Source: CAD feature listing. Evaluate the final solid. Frame: model axes, mm. Round coordinates to 2 decimals unless told otherwise and drop trailing zeros. Loops run counter-clockwise (first coordinate to the right, second up) from the corner with the lowest first, then second, coordinate; pieces in that order, holes last. Notation, with made-up numbers: M 62.5,-1 L 108.5,-1 A27 ccw 108.5,23 Z; hole C -38.5,-25.5 d9. An arc over 180 degrees is marked long. Answer as a JSON object with one key per item and string values.
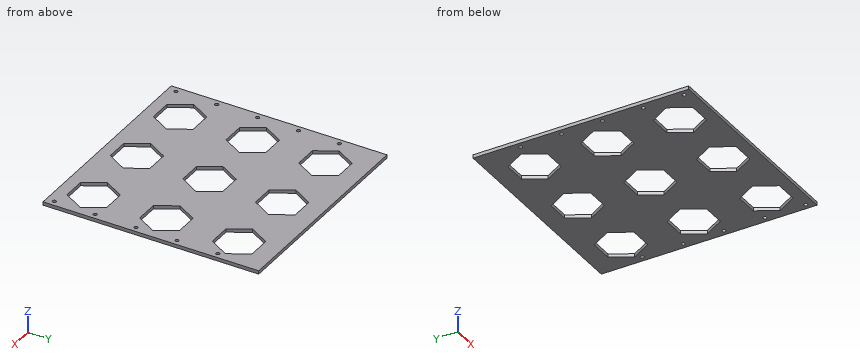
from build123d import *

# Parameters (mm, degrees)
SKETCH_1_W          = 190
SKETCH_1_H          = 190
EXTRUDE_1_DEPTH     = 3
CUT_EXTRUDE_1_DEPTH = 3
SKETCH_3_R          = 1.6
CUT_EXTRUDE_2_DEPTH = 10


with BuildPart() as part:
    # 草图1 → 凸台-拉伸1 (new body)
    with BuildSketch(Plane.XY):
        with Locations((95, -95)):
            Rectangle(SKETCH_1_W, SKETCH_1_H)
    extrude(amount=EXTRUDE_1_DEPTH)

    # 草图2 → 切除-拉伸1 (cut)
    with BuildSketch(Plane.XY.offset(3)):
        Polygon((54.207259422, -34), (44.103629711, -16.5), (23.896370289, -16.5), (13.792740578, -34), (23.896370289, -51.5), (44.103629711, -51.5), align=None)
        Polygon((108.103629711, -16.5), (87.896370289, -16.5), (77.792740578, -34), (87.896370289, -51.5), (108.103629711, -51.5), (118.207259422, -34), align=None)
        Polygon((172.103629711, -16.5), (151.896370289, -16.5), (141.792740578, -34), (151.896370289, -51.5), (172.103629711, -51.5), (182.207259422, -34), align=None)
        Polygon((108.103629711, -80.5), (87.896370289, -80.5), (77.792740578, -98), (87.896370289, -115.5), (108.103629711, -115.5), (118.207259422, -98), align=None)
        Polygon((172.103629711, -80.5), (151.896370289, -80.5), (141.792740578, -98), (151.896370289, -115.5), (172.103629711, -115.5), (182.207259422, -98), align=None)
        Polygon((108.103629711, -144.5), (87.896370289, -144.5), (77.792740578, -162), (87.896370289, -179.5), (108.103629711, -179.5), (118.207259422, -162), align=None)
        Polygon((172.103629711, -144.5), (151.896370289, -144.5), (141.792740578, -162), (151.896370289, -179.5), (172.103629711, -179.5), (182.207259422, -162), align=None)
        Polygon((44.103629711, -80.5), (23.896370289, -80.5), (13.792740578, -98), (23.896370289, -115.5), (44.103629711, -115.5), (54.207259422, -98), align=None)
        Polygon((44.103629711, -144.5), (23.896370289, -144.5), (13.792740578, -162), (23.896370289, -179.5), (44.103629711, -179.5), (54.207259422, -162), align=None)
    extrude(amount=-CUT_EXTRUDE_1_DEPTH, mode=Mode.SUBTRACT)

    # 草图3 → 切除-拉伸2 (cut)
    with BuildSketch(Plane.XY.offset(3)):
        with Locations((5, -75)):
            Circle(SKETCH_3_R)
        with Locations((185, -75)):
            Circle(SKETCH_3_R)
        with Locations((5, -111)):
            Circle(SKETCH_3_R)
        with Locations((185, -111)):
            Circle(SKETCH_3_R)
        with Locations((5, -147)):
            Circle(SKETCH_3_R)
        with Locations((185, -147)):
            Circle(SKETCH_3_R)
        with Locations((5, -183)):
            Circle(SKETCH_3_R)
        with Locations((185, -183)):
            Circle(SKETCH_3_R)
        with Locations((5, -39)):
            Circle(SKETCH_3_R)
        with Locations((185, -39)):
            Circle(SKETCH_3_R)
    extrude(amount=-CUT_EXTRUDE_2_DEPTH, mode=Mode.SUBTRACT)


solid = part.part
Item 1: Section B-B on y = -105.5. Return the cut outline in (x, z), then the cut area to 3 significant figures.
Answer sheet:
{"outline": "M 0,0 L 18.12,0 L 18.12,3 L 0,3 Z; M 49.88,0 L 82.12,0 L 82.12,3 L 49.88,3 Z; M 113.88,0 L 146.12,0 L 146.12,3 L 113.88,3 Z; M 177.88,0 L 190,0 L 190,3 L 177.88,3 Z", "area": "284 mm²"}
Item 2: Section A-A on x = 28. Return the cut outline in (y, z), then the cut area to 3 significant figures.
Answer sheet:
{"outline": "M -190,0 L -179.5,0 L -179.5,3 L -190,3 Z; M -144.5,0 L -115.5,0 L -115.5,3 L -144.5,3 Z; M -80.5,0 L -51.5,0 L -51.5,3 L -80.5,3 Z; M -16.5,0 L 0,0 L 0,3 L -16.5,3 Z", "area": "255 mm²"}
Item 3: Line query: probe 1 along X at (y, z) = (-75, 1.35); probe 2 along Y at (x, z) = (41, 1.75); probe 3 along Y at (x, z) = (185, 1.5). Output: solid intervals per line, ascending. Write a range as from..to.
Answer sheet:
{"probe 1": "x = 0..3.4, 6.6..183.4, 186.6..190", "probe 2": "y = -190..-179.5, -144.5..-115.5, -80.5..-51.5, -16.5..0", "probe 3": "y = -190..-184.6, -181.4..-148.6, -145.4..-112.6, -109.4..-76.6, -73.4..-40.6, -37.4..0"}
Item 4: Contact query for flat-ended pins moving along their axis: pin 1 Ø3.5 at (x, y) = (185, -111) entering from -Z; pin 2 Ø3 at (x, y) = (185, -147) entering from +Z. Output: stop coordinate, or through.
Answer sheet:
{"pin 1": "stops at z = 0", "pin 2": "passes through"}
Item 5: Section C-C on z = 2.3. Give the number of separate pieces and of enclosed holes in the cut face, then the cut area to 3 significant figures.
Answer sheet:
{"separate pieces": "1", "enclosed holes": "19", "area": "26,500 mm²"}
